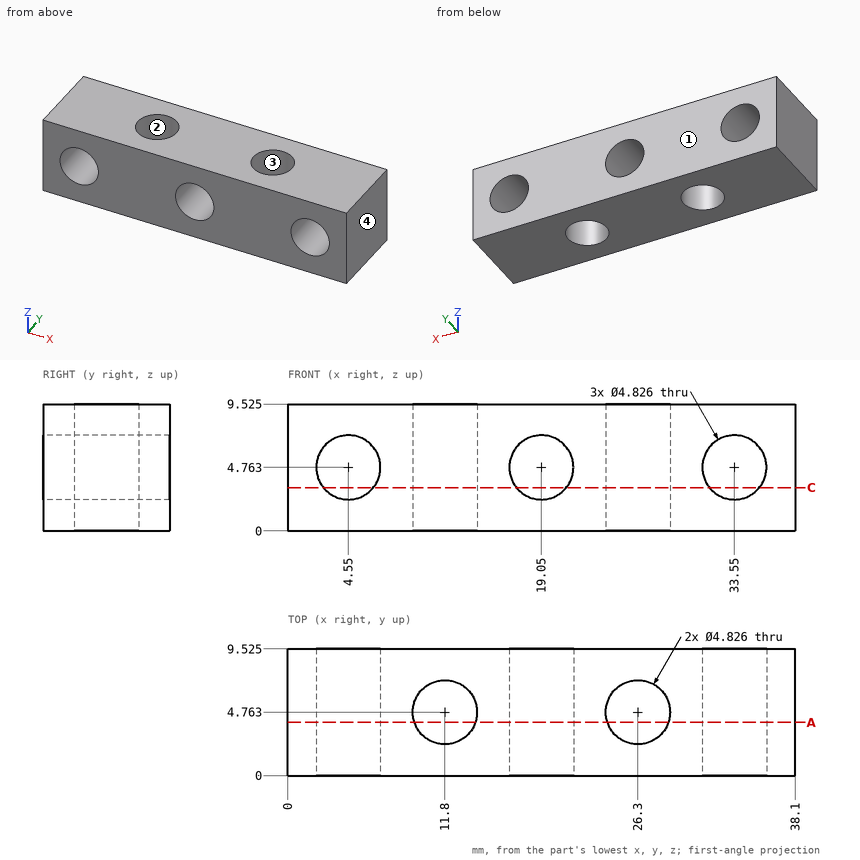
Design review of the part shown in the three views and the two pictorial views. Dimensions are in mm from the part's minimum x, y and z. Coordinates: 2 decimals unless noted, no trailing zeros. Order: outer loops, then holes, each group sorted by start corner. A loop starts at its lowest first (then second) coordinate and runs counter-clockwise, first axis right, second up.
Item 1: For line 1 (Y direction, x = 12, z = 3.5) (1 decimal); line 2 (X direction, y = 6, z = 1.75); line 3 (X direction, y = 2.75, z = 9) (1 decimal), list the stretches that pass through material, from the lowest coordinate up.
Item 2: The part is to be moulded in two halves that separate along Y. For the marked faces 1, 2, 3 and 4, say which applies: pulls with the +Y half, pulls with the -Y half, needs draft (parallel to the pull), parting line crosses it, or undercut.
Item 3: Take a section at C-C, the plane z = 3.25. Write out the cut boundary in (x, y) (1 decimal), then the cut area to 3 significant figures.
Item 4: Take a section at A-A, the plane y = 4. Count the separate pieces of the cut face and the enclosed holes in it, then the cut area to 3 significant figures.
Item 5: For pin 1 Ø3 at (y, z) = (1.5, 4.5) entering from -X, flat-tipped, find the tip position at first contact; note if it passes through.
The answers:
1. line 1: y = 0 to 2.4, 7.2 to 9.5
1. line 2: x = 0 to 9.73, 13.87 to 24.23, 28.37 to 38.1
1. line 3: x = 0 to 10.5, 13.1 to 25, 27.6 to 38.1
2. face 1: pulls with the +Y half
2. face 2: undercut
2. face 3: undercut
2. face 4: needs draft
3. outline: (0, 0) - (2.7, 0) - (2.7, 9.5) - (0, 9.5) - close; (6.4, 0) - (17.2, 0) - (17.2, 9.5) - (6.4, 9.5) - close; (20.9, 0) - (31.7, 0) - (31.7, 9.5) - (20.9, 9.5) - close; (35.4, 0) - (38.1, 0) - (38.1, 9.5) - (35.4, 9.5) - close; hole circle Ø4.8 at (11.8, 4.8); hole circle Ø4.8 at (26.3, 4.8)
3. area: 219 mm2
4. separate pieces: 3
4. enclosed holes: 3
4. area: 221 mm2
5. pin 1: stops at x = 0
